Model file for the job. Use its own axes, mm. Face numbers are marked on the shaded views. Round coordinates to 2 decimals unless told otherwise and drop trailing zeros. Order: outer loops, then holes, each group sorted by start corner. A loop starts at its lowest first (then second) coordinate and runs counter-clockwise, first axis right, second up. Notation, with made-up numbers: (31, -33) -> (70, -33) arc R16 ccw to (70, -23) -> close; hole circle Ø8 at (-35, 85). An arc over 180 degrees is marked (long way). Use CSV: the item, a comma, the result in double quotes.
Autodesk Inventor part; units mm, degrees
ref_plane "YZ Plane" through (0, 0, 0) normal (1, 0, 0) x (0, 1, 0)
ref_plane "XZ Plane" through (0, 0, 0) normal (0, 1, 0) x (-1, 0, 0)
ref_plane "XY Plane" through (0, 0, 0) normal (0, 0, 1) x (1, 0, 0)
sketch "Sketch1 - base" plane through (0, 0, 0) normal (0, 0, 1) x (1, 0, 0)
  circle A0 centre (0, 0) radius 3.5
  line L0 (-3.5, 0) -> (-3.5, 10)
  line L1 (-3.5, 10) -> (3.5, 10)
  line L2 (3.5, 10) -> (3.5, 0)
  dimension "d0" = 7
  dimension "d1" = 10
extrude "Extrusion1" add sketch "Sketch1 - base" along normal blind 4
sketch "Sketch2 - axle_hole" plane through (0, 0, 0) normal (0, 0, -1) x (-1, 0, 0)
  circle A0 centre (0, 0) radius 2.275
  arc A1 (-2.1959, 0.5948) -> (-2.275, 0) centre (-2.256, 0.3001) ccw
  line L0 (-2.256, 0.3001) -> (-2.5544, 0.3398) construction
  arc A2 (-2.2722, -0.1129) -> (-2.1637, -0.703) centre (-2.2383, -0.4117) ccw
  arc A3 (-2.1261, -0.8095) -> (-1.8405, -1.3372) centre (-2.0015, -1.0832) ccw
  arc A4 (-1.7719, -1.4269) -> (-1.3372, -1.8405) centre (-1.5688, -1.6487) ccw
  arc A5 (-1.2442, -1.9046) -> (-0.703, -2.1637) centre (-0.9826, -2.0528) ccw
  arc A6 (-0.5948, -2.1959) -> (0, -2.275) centre (-0.3001, -2.256) ccw
  arc A7 (0.1129, -2.2722) -> (0.703, -2.1637) centre (0.4117, -2.2383) ccw
  arc A8 (0.8095, -2.1261) -> (1.3372, -1.8405) centre (1.0832, -2.0015) ccw
  arc A9 (1.4269, -1.7719) -> (1.8405, -1.3372) centre (1.6487, -1.5688) ccw
  arc A10 (1.9046, -1.2442) -> (2.1637, -0.703) centre (2.0528, -0.9826) ccw
  arc A11 (2.1959, -0.5948) -> (2.275, 0) centre (2.256, -0.3001) ccw
  arc A12 (2.2722, 0.1129) -> (2.1637, 0.703) centre (2.2383, 0.4117) ccw
  arc A13 (2.1261, 0.8095) -> (1.8405, 1.3372) centre (2.0015, 1.0832) ccw
  arc A14 (1.7719, 1.4269) -> (1.3372, 1.8405) centre (1.5688, 1.6487) ccw
  arc A15 (1.2442, 1.9046) -> (0.703, 2.1637) centre (0.9826, 2.0528) ccw
  arc A16 (0.5948, 2.1959) -> (0, 2.275) centre (0.3001, 2.256) ccw
  arc A17 (-0.1129, 2.2722) -> (-0.703, 2.1637) centre (-0.4117, 2.2383) ccw
  arc A18 (-0.8095, 2.1261) -> (-1.3372, 1.8405) centre (-1.0832, 2.0015) ccw
  arc A19 (-1.4269, 1.7719) -> (-1.8405, 1.3372) centre (-1.6487, 1.5688) ccw
  arc A20 (-1.9046, 1.2442) -> (-2.1637, 0.703) centre (-2.0528, 0.9826) ccw
  point P0 (-2.2722, -0.1129)
  point P1 (-2.1261, -0.8095)
  point P2 (-1.8405, -1.3372)
  point P3 (-1.3372, -1.8405)
  point P4 (-1.2442, -1.9046)
  point P5 (-0.5948, -2.1959)
  point P6 (0, -2.275)
  point P7 (0.1129, -2.2722)
  point P8 (0.8095, -2.1261)
  point P9 (1.3372, -1.8405)
  point P10 (1.4269, -1.7719)
  point P11 (1.8405, -1.3372)
  point P12 (1.9046, -1.2442)
  point P13 (2.1637, -0.703)
  point P14 (2.1959, -0.5948)
  point P15 (2.275, 0)
  point P16 (2.2722, 0.1129)
  point P17 (2.1637, 0.703)
  point P18 (2.1261, 0.8095)
  point P19 (1.8405, 1.3372)
  point P20 (1.7719, 1.4269)
  point P21 (1.3372, 1.8405)
  point P22 (1.2442, 1.9046)
  point P23 (0.703, 2.1637)
  point P24 (0.5948, 2.1959)
  point P25 (0, 2.275)
  point P26 (-0.1129, 2.2722)
  point P27 (-0.703, 2.1637)
  point P28 (-0.8095, 2.1261)
  point P29 (-1.3372, 1.8405)
  point P30 (-1.4269, 1.7719)
  point P31 (-1.8405, 1.3372)
  point P32 (-1.9046, 1.2442)
  point P33 (-2.1637, 0.703)
  dimension "d4" = 4.55
  dimension "d16" = 0.6
  dimension "d17" = 0.301
  dimension "d20" = 360
extrude "Extrusion2" cut sketch "Sketch2 - axle_hole" against normal blind 2
sketch "Sketch3 - screw_hole" plane through (0, 0, 0) normal (0, 0, -1) x (-1, 0, 0)
  circle A0 centre (0, 0) radius 1.1
  dimension "d12" = 2.2
extrude "Extrusion3" cut sketch "Sketch3 - screw_hole" against normal blind 4
fillet "Fillet1" radius 1.5 2 edges at (3.5, 10, 2) (-3.5, 10, 2)
properties part number "Motor Axle Fitting Test"
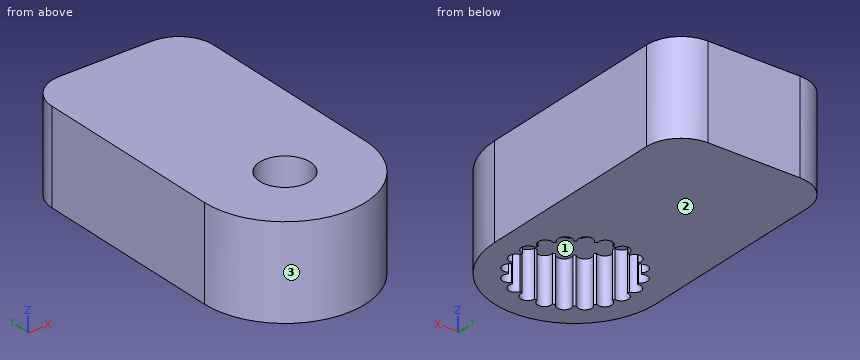
Q1. Probe line 1 along Y through (x, z) = (0, 2.6); line 2 along Y through (x, z) = (0.75, 0.6); line 3 along Z through (x, y) = (-0.5, 2.25). List the from-to ranges inside material, lowest first.
From the geometry:
line 1,"y = -3.5 to -1.1, 1.1 to 10"
line 2,"y = -3.42 to -2.24, 2.15 to 10"
line 3,"z = 2 to 4"
Q2. Cut at B-B (x = 2.75). Give the cut face in (y, z).
From the geometry:
outline,"(-2.17, 0) -> (9.8, 0) -> (9.8, 4) -> (-2.17, 4) -> close"
Q3. Pin check, flat tips, straight feed: pin 1 (2 mm diameter, centred on x = 2, z = 2, fed in from -Y); pin 2 (1.3 mm diameter, centred on x = 0, y = 0, fed in from -Z). Stop position of each tip, or through.
From the geometry:
pin 1,"stops at y = -3.35"
pin 2,"passes through"
Q4. Mould opens along X. For the marked faces 1, 2 and 3 say: +X half, -X half, draft (parallel to the pull), parting line (faces both ways), or undercut.
From the geometry:
face 1,"undercut"
face 2,"draft"
face 3,"parting line"
Q5. Cut at A-A (z = 3.3). Give the cut face in (x, y).
From the geometry:
outline,"(-3.5, 0) arc R3.5 ccw to (3.5, 0) -> (3.5, 8.5) arc R1.5 ccw to (2, 10) -> (-2, 10) arc R1.5 ccw to (-3.5, 8.5) -> close; hole circle Ø2.2 at (0, 0)"
